Check sheet for the modelled part. Datum: model origin and axes. Units: mm. Coordinates: 2 decimals unless noted, no trailing zeros. Order: outer loops, then holes, each group sorted by start corner. A loop starts at its lowest first (then second) coordinate and runs counter-clockwise, first axis right, second up.
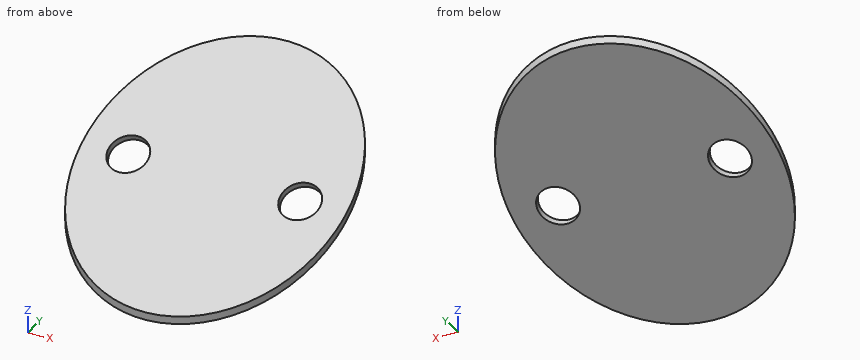
from build123d import *

# Parameters (mm, degrees)
F0_R      = 15.875
F1_DEPTH  = 25.4
F5_R      = 28.0073181772
F6_DEPTH  = 25.4
F7_R      = 26.7212354085
F8_DEPTH  = 25.4
F9_R      = 2.3876
F10_DEPTH = 25.4


with BuildPart() as f1:
    # F0 (on Top) → F1 (new body)
    with BuildSketch(Plane.XY):
        Circle(F0_R)
    extrude(amount=F1_DEPTH)

    # F5 (on offset) → F6 (cut)
    with BuildSketch(Plane(origin=(0, -5.645975072, 10.6185347405), x_dir=(1, 0, 0), z_dir=(0, -0.4694715628, 0.8829475929))):
        Circle(F5_R)
    extrude(amount=F6_DEPTH, mode=Mode.SUBTRACT)

    # F7 (on line) → F8 (cut)
    with BuildSketch(Plane(origin=(0, -5.2643885857, 9.900874937), x_dir=(1, 0, 0), z_dir=(0, -0.4694715628, 0.8829475929))):
        with Locations((-3.1001365278, 4.3183793314)):
            Circle(F7_R)
    extrude(amount=-F8_DEPTH, mode=Mode.SUBTRACT)

    # F9 (on line) → F10 (cut)
    with BuildSketch(Plane(origin=(0, -5.2643885857, 9.900874937), x_dir=(1, 0, 0), z_dir=(0, -0.4694715628, 0.8829475929))):
        with Locations((-10.3505, 6.1972388474)):
            Circle(F9_R)
        with Locations((10.3505, 6.1972388474)):
            Circle(F9_R)
    extrude(amount=F10_DEPTH, mode=Mode.SUBTRACT)


solid = f1.part
(1) Cross-section at C-C (y = -1). Count the separate pieces of the cut face and the enclosed holes in it, and give its area (3 significant figures).
Filled in:
separate pieces: 3
enclosed holes: 0
area: 21.5 mm2
(2) Go/stop test with flat-tipped pins: P1, Ø1.5, axis at x = -7, y = 2, coming from the +Z side; P2, Ø6, axis at x = -7.5, z = 19, coming from the +Y side; P3, Ø5, axis at y = 10, z = 16.5, coming from the -X side; P4, Ø1, axis at y = 2.5, z = 16, coming from the -X side. Record where each tip stops, or that it passes through.
Filled in:
P1: stops at z = 15.08
P2: stops at y = 15.06
P3: stops at x = -13.99
P4: passes through
(3) Cross-section at A-A (x = -12). Enter the section's corners in (y, z).
Filled in:
outline: (-10.39, 7.17) - (-1.32, 12) - (-1.7, 12.72) - (-10.39, 8.09) - close; (1.35, 14.34) - (1.73, 13.62) - (10.39, 18.23) - (10.39, 19.15) - close
(4) Cross-section at D-D (z = 7). Enter the section's corners in (x, y) (3 decimals).
Filled in:
outline: (-11.709, -10.72) arc R15.875 ccw to (-9.848, -12.451) - (9.848, -12.451) arc R15.875 ccw to (11.709, -10.72) - close
(5) Thickness scan on probe 1 along Y at (x, z) = (-12, 14.75); probe 2 along Z at (x, y) = (0, -11); probe 3 along Y at (x, z) = (6, 11). Record the ranges inside material, lowest first.
Filled in:
probe 1: y = 2.12 to 3.86
probe 2: z = 6.85 to 7.77
probe 3: y = -4.93 to -3.2
(6) Cross-section at B-B (x = 0). Enter the section's corners in (y, z) (3 decimals).
Filled in:
outline: (-15.875, 4.259) - (15.875, 21.141) - (15.875, 22.061) - (-15.875, 5.18) - close
